Study the drawing (mm; zero at the part's minimum x, y, z) and answer. A direction names the side the tool comes from. Coordinates: 2 decimals unless noted, no trailing zeros. Write each loop counter-clockwise with the first axis right and the second up, starting at its lowest first coordinate (ties: lowest second). Pieces come first, ordered by that corner, then holes. Notation, with made-up numbers: M -1.75,54 L 41.25,54 A7 cw 41.25,58 Z; hole C -12,81.25 d5. An arc over 180 degrees is marked long. Answer as CSV lines item,"result". Start each with the question number.
(1) A cutting plane is placed at D-D on x = 97. Give the vertices of the cut face in (y, z) (1 decimal), then the cut area to 3 significant figures.
(2) Find the intervals of material crossed by L1, parallel to Y at x = 58, z = 7.5 (1 decimal); L2, parallel to X at y = 79.5, z = 14.5 (1 decimal); L3, parallel to Z at x = 71, y = 71, in increasing order. Write a range as [from, to].
(3) The mould has two halves that part along Y. Classify the marked faces 4, 5 and 6: released by +Y, released by -Y, zero draft, split by the parting line, or undercut.
(4) A cutting plane is placed at C-C on z = 54.5. Give the vertices of the cut face in (x, y) (1 decimal), then the cut area to 3 significant figures.
(5) A cutting plane is placed at A-A on y = 38. Give the vertices of the cut face in (x, z).
(6) A cutting plane is placed at B-B on x = 72. Give the vertices of the cut face in (y, z), then the cut area to 3 significant figures.
(7) Flat-ended cylindrical pins translate along their axes: P1, Ø1.5, axis at y = 13, z = 49.5, coming from the +X side; P2, Ø8, axis at y = 23.5, z = 13, coming from the -X side; P3, Ø1, axis at x = 54.5, z = 7, coming from the -Y side; P4, Ø5, axis at x = 62.6, y = 62.6, coming from the -Z side. Find the tip coordinate at first contact, or state that the pin passes through.
(8) For the marked faces 1, 2 and 3, determine the directions among +Z, -Z, +X, -X, +Y, -Y from which every point of the face is accessible in a straight line to the end or side of a thin tool.
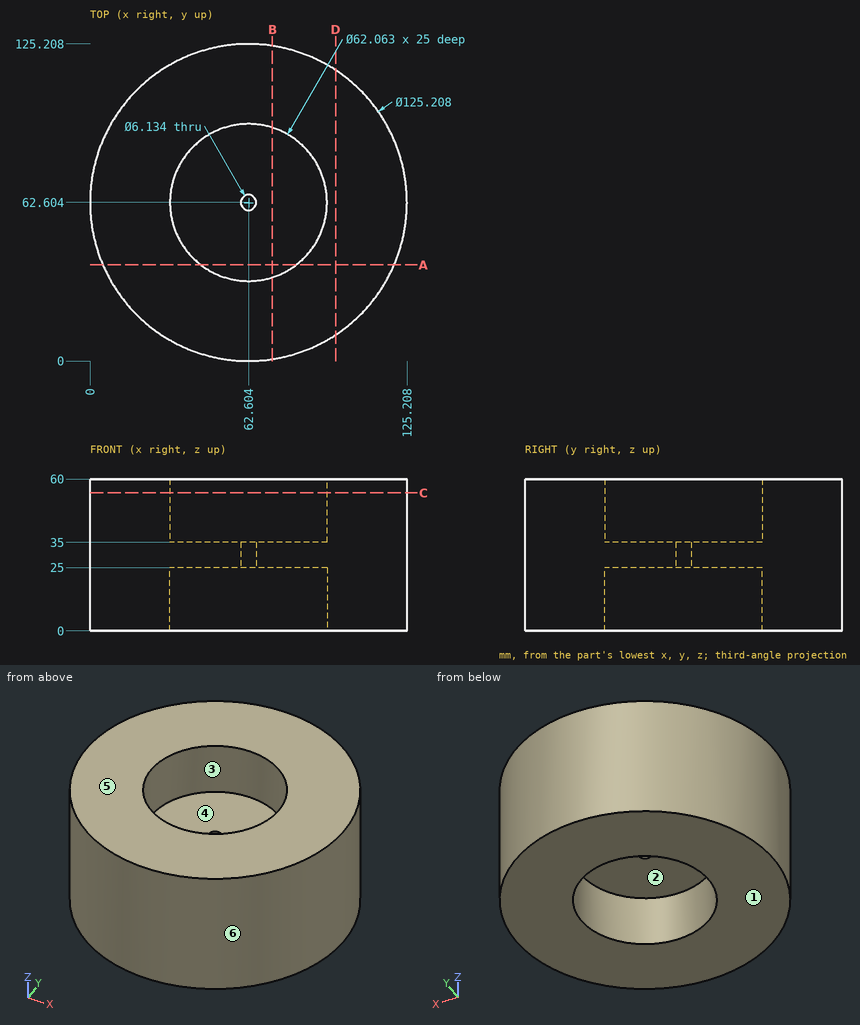
Here are the results:
1,outline,"M 10.3,0 L 114.9,0 L 114.9,60 L 10.3,60 Z"
1,area,"6,280 mm^2"
2,L1,"y = [0.2, 31.9], [93.3, 125]"
2,L2,"x = [2.3, 36.6], [88.6, 122.9]"
2,L3,"z = [25, 35]"
3,face 4,"undercut"
3,face 5,"zero draft"
3,face 6,"split by the parting line"
4,outline,"C 62.6,62.6 d125.2; hole C 62.6,62.6 d62.1"
4,area,"9,290 mm^2"
5,outline,"M 5.04,0 L 43.69,0 L 43.69,25 L 81.51,25 L 81.51,0 L 120.17,0 L 120.17,60 L 81.51,60 L 81.51,35 L 43.69,35 L 43.69,60 L 5.04,60 Z"
6,outline,"M 0.71,0 L 33.03,0 L 33.03,25 L 92.18,25 L 92.18,0 L 124.5,0 L 124.5,60 L 92.18,60 L 92.18,35 L 33.03,35 L 33.03,60 L 0.71,60 Z"
6,area,"4,470 mm^2"
7,P1,"stops at x = 101.75"
7,P2,"stops at x = 10.77"
7,P3,"stops at y = 0.46"
7,P4,"passes through"
8,face 1,"-Z, +X, -X, +Y, -Y"
8,face 2,"-Z"
8,face 3,"+Z"
